The model under review builds one solid part; all positions refer to its coordinate system, in mm. Face numbers are marked on the shaded views. A direction names the side the tool comes from. Coordinates: 2 decimals unless noted, no trailing zeros. Order: outer loops, then holes, each group sorted by start corner. A loop starts at its lowest first (then second) coordinate and runs counter-clockwise, first axis right, second up. Notation, with made-up numbers: M 28,-29.5 L 79,-29.5 A26 cw 79,-4.5 Z; hole C -11.75,76 d1. An arc over 180 degrees is marked long. One line per item, written item: value.
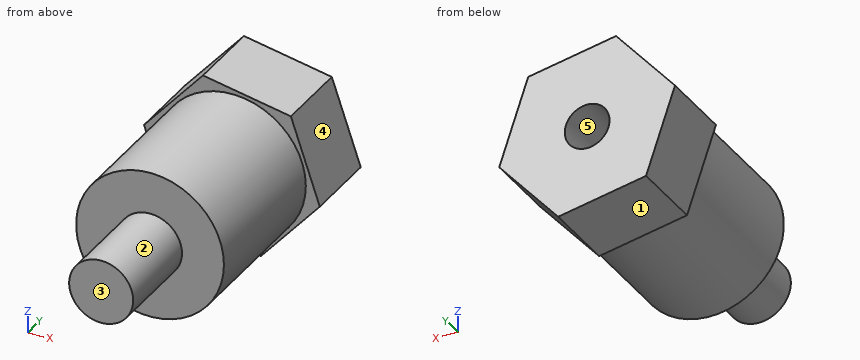
```python
from build123d import *

# Parameters (mm, degrees)
BOSS_EXTRUDE1_DEPTH = 6
SKETCH2_R           = 5.775
BOSS_EXTRUDE2_DEPTH = 18
SKETCH3_R           = 2.5
BOSS_EXTRUDE3_DEPTH = 7.16
SKETCH4_R           = 1.75
CUT_EXTRUDE1_DEPTH  = 10


with BuildPart() as part:
    # Sketch1 → Boss-Extrude1 (new body)
    with BuildSketch(Plane(origin=(0, 0, 0), x_dir=(1, 0, 0), z_dir=(0, 1, 0))):
        Polygon((4.605908032, -5.271205859), (6.867952198, 1.353230434), (2.262044166, 6.624436292), (-4.605908032, 5.271205859), (-6.867952198, -1.353230434), (-2.262044166, -6.624436292), align=None)
    extrude(amount=BOSS_EXTRUDE1_DEPTH)

    # Sketch2 → Boss-Extrude2 (add)
    with BuildSketch(Plane(origin=(0, 6, 0), x_dir=(1, 0, 0), z_dir=(0, 1, 0))):
        Circle(SKETCH2_R)
    extrude(amount=-BOSS_EXTRUDE2_DEPTH)

    # Sketch3 → Boss-Extrude3 (add)
    with BuildSketch(Plane.XZ.offset(12)):
        Circle(SKETCH3_R)
    extrude(amount=BOSS_EXTRUDE3_DEPTH)

    # Sketch4 → Cut-Extrude1 (cut)
    with BuildSketch(Plane(origin=(0, 6, 0), x_dir=(1, 0, 0), z_dir=(0, 1, 0))):
        Circle(SKETCH4_R)
    extrude(amount=-CUT_EXTRUDE1_DEPTH, mode=Mode.SUBTRACT)


solid = part.part
```
(1) We need section C-C, the plane z = 0. State the section outline as (x, y) points (3 decimals), plus the area to 3 significant figures.
Geometry results:
outline: M -6.406,0 L -5.775,0 L -5.775,-12 L -2.5,-12 L -2.5,-19.16 L 2.5,-19.16 L 2.5,-12 L 5.775,-12 L 5.775,0 L 6.406,0 L 6.406,6 L 1.75,6 L 1.75,-4 L -1.75,-4 L -1.75,6 L -6.406,6 Z
area: 216 mm2
(2) We need section A-A, the plane x = 0. State the section outline as (y, z) points (3 decimals).
Geometry results:
outline: M -19.16,-2.5 L -12,-2.5 L -12,-5.775 L 0,-5.775 L 0,-6.179 L 6,-6.179 L 6,-1.75 L -4,-1.75 L -4,1.75 L 6,1.75 L 6,6.179 L 0,6.179 L 0,5.775 L -12,5.775 L -12,2.5 L -19.16,2.5 Z
(3) Tool access review of the marked faces 1 and 2: name each direction out of +Z, -Z, +X, -X, +Y, -Y from which nothing blocks a thin tool from reaching the whole face with its end or side.
Geometry results:
face 1: -Z, -X, +Y, -Y
face 2: -Y
(4) Mouldability with a two-part tool opening along X and no side actions: class the marked faces 3, 4 and 5 as +X half, -X half, draft (parallel to the pull), parting line (faces both ways), or undercut.
Geometry results:
face 3: draft
face 4: +X half
face 5: undercut
(5) We need section B-B, the plane y = -0.5. State the section outline as (x, z) points (3 decimals), plus the area to 3 significant figures.
Geometry results:
outline: C 0,0 d11.55; hole C 0,0 d3.5
area: 95.2 mm2
(6) For L1, parallel to X at y = -0.5, z = 0 (3 decimals); L2, parallel to Y at x = 4.25, z = -2.25; L3, parallel to X at y = 3.75, z = 0, list the stretches that pass through material, from the lowest coordinate up.
Geometry results:
L1: x = -5.775 to -1.75, 1.75 to 5.775
L2: y = -12 to 6
L3: x = -6.41 to -1.75, 1.75 to 6.41
(7) Insertion check: pin 1 Ø4 at (x, z) = (-2.5, 2) entering from -Y. The pin has a flat end and moves straight along its axis. Give the tip position at first contact, or say it passes through.
Geometry results:
pin 1: stops at y = -19.16
(8) We need section D-D, the plane y = -14.25. State the section outline as (x, z) points, plus the area to 3 significant figures.
Geometry results:
outline: C 0,0 d5
area: 19.6 mm2
